```python
from build123d import *

# Parameters (mm, degrees)
F1_DEPTH = 50
F3_DEPTH = 50.0010001
F4_R     = 16.0196182497
F5_DEPTH = 37.7
F6_R     = 14.0015155941
F7_DEPTH = 63


with BuildPart() as f1:
    # F0 (on Front) → F1 (new body)
    with BuildSketch(Plane.XZ):
        with BuildLine():
            add(Edge.make_bspline(
                [(-24.9009096901, 27.8132260291), (-15.2719138126, 25.0041245055), (0.0685505815, 19.3712880215), (15.1674460028, 23.7765369464), (25.1386704972, 26.9907502037)],
                knots=[0, 0, 0, 0, 0.4997319812, 1, 1, 1, 1], degree=3))
            Line((-24.9009096901, 27.8132260291), (-30.8519195794, 31.2922782778))
            ThreePointArc((-30.8519195794, 31.2922782778), (-31.6756477165, 29.0091165086), (-33.2958245412, 27.2018028212))
            Line((-33.2958245412, 27.2018028212), (-25.9555131602, 21.8371527458))
            add(Edge.make_bspline(
                [(-25.9555131602, 21.8371527458), (-22.7845221536, 13.488346606), (-17.3288820912, 0.0516611316), (-22.1761950436, -11.8040839548), (-25.4937373126, -18.8575223359)],
                knots=[0, 0, 0, 0, 0.5176887267, 1, 1, 1, 1], degree=3))
            Line((-25.4937373126, -18.8575223359), (-34.3650811811, -24.4237805158))
            ThreePointArc((-34.3650811811, -24.4237805158), (-32.3719868097, -26.6370212042), (-31.6072761212, -29.5155758903))
            Line((-31.6072761212, -29.5155758903), (-23.0260640383, -24.6824789792))
            add(Edge.make_bspline(
                [(-23.0260640383, -24.6824789792), (-14.7885032622, -22.1197617809), (-0.0436946051, -14.9712963525), (16.3980588143, -23.2713009768), (25.1386702767, -26.1990372013)],
                knots=[0, 0, 0, 0, 0.4877897865, 1, 1, 1, 1], degree=3))
            Line((25.1386702767, -26.1990372013), (28.7010856366, -28.4007272488))
            ThreePointArc((28.7010856366, -28.4007272488), (29.5711101683, -25.4013798938), (31.7657258985, -23.1795137775))
            Line((31.7657258985, -23.1795137775), (25.1386702897, -18.8575223359))
            add(Edge.make_bspline(
                [(27.0089022596, 21.8371527458), (24.067082439, 13.1959431089), (15.6637973801, 0.5258679424), (22.3337226969, -12.2190983175), (25.1386702897, -18.8575223359)],
                knots=[0, 0, 0, 0, 0.5199533553, 1, 1, 1, 1], degree=3))
            Line((27.0089022596, 21.8371527458), (32.2177472852, 26.0263319884))
            ThreePointArc((32.2177472852, 26.0263319884), (30.448037412, 27.4639143113), (29.311723773, 29.440605305))
            Line((29.311723773, 29.440605305), (25.1386704972, 26.9907502037))
        make_face()
    extrude(amount=F1_DEPTH)

    # F2 (on face) → F3 (cut, through all)
    with BuildSketch(Plane.XZ.offset(50)):
        with BuildLine():
            add(Edge.make_bspline(
                [(-25.9555131602, 21.8371527458), (-22.7845221536, 13.488346606), (-17.3288820912, 0.0516611316), (-22.1761950436, -11.8040839548), (-25.4937373126, -18.8575223359)],
                knots=[0, 0, 0, 0, 0.5176887267, 1, 1, 1, 1], degree=3))
            ThreePointArc((-25.4937373126, -18.8575223359), (-14.3192522827, 1.6192357189), (-25.9555131602, 21.8371527458))
        make_face()
    extrude(amount=-F3_DEPTH, mode=Mode.SUBTRACT)

    # F4 (on Front) → F5 (cut)
    with BuildSketch(Plane.XZ):
        with Locations((22.9763758397, 0.8501823597)):
            Circle(F4_R)
    extrude(amount=-F5_DEPTH, mode=Mode.SUBTRACT)

    # F6 (on Front) → F7 (cut)
    with BuildSketch(Plane.XZ):
        with Locations((-1.843900617, 21.1695458569)):
            Circle(F6_R)
    extrude(amount=-F7_DEPTH, mode=Mode.SUBTRACT)


solid = f1.part
```
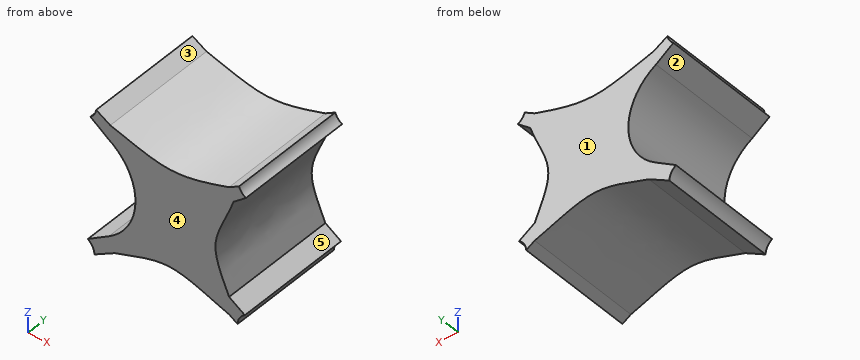
Source: CAD feature listing. Evaluate the final solid. Frame: model axes, mm. Face numbers are marked on the shaded views. A direction names the side the tool comes from. Give positions to 0.01 mm unless a question says otherwise; leave off trailing zeros. Put each result on its own line as item: value.
Q1. Line query: probe 1 along X at (y, z) = (-4, 29); probe 2 along Z at (x, y) = (-30, -34); probe 3 along Z at (x, y) = (8, -26.5). Output: solid intervals per line, ascending. Write a range as [from, to].
Response values:
probe 1: x = [-31.68, -26.93], [28.56, 29.49]
probe 2: z = [-28.61, -21.68], [24.79, 30.79]
probe 3: z = [-20.14, 22.4]
Q2. Pin query (flat end, axial travel): P1, Ø1, axis at y = -6.5, z = 19.5, coming from the -X side; P2, Ø10, axis at x = -16.5, y = -39.5, coming from the -Z side; P3, Ø1, axis at y = -10.5, z = -7.5, coming from the +X side. Return the tip coordinate at first contact, or that it passes through.
Response values:
P1: stops at x = -23.3
P2: stops at z = -24.19
P3: stops at x = 20.7
Q3. Reachability of the marked faces 1 and 2 from +Z, -Z, +X, -X, +Y, -Y: full face, straight path, thin tool, end or side. Return the list, or none.
Response values:
face 1: +Z, -Z, +X, -X, +Y
face 2: -X, +Y, -Y
Q4. Mould query, pull axis Z, two halves, no side actions, for the marked faces 3, 4 and 5. Classes: released by +Z, released by -Z, zero draft, split by the parting line, or undercut.
Response values:
face 3: released by +Z
face 4: zero draft
face 5: undercut
